Input: part model. Units: mm. Frame: model coordinates. A direction names the side the tool comes from. Coordinates: 2 decimals unless noted, no trailing zeros. Write each loop counter-clockwise with the first axis right and the second up, starting at its lowest first coordinate (ties: lowest second). Pieces come first, ordered by that corner, then holes. Notation, with made-up numbers: M 72,75 L 84,75 A16 ccw 84,105 Z; hole C 55.5,5.25 d10. An arc over 180 degrees is marked long. Write each question's results on one line, items separated by ' | '. Start each with the question number.
1. Ray query, probe 1 along Y at (x, z) = (30, 9.2); probe 2 along Y at (x, z) = (-1.7, 0.8); probe 3 along X at (y, z) = (-19, 0.75). Return the intervals inside material, ascending.
2. Section query A-A, the plane x = 12. Output: boundary loops of the cut face in (y, z).
3. Pull-direction query (Y, two-part tool) for faces 1 (the flat face through (-1, 17, 10)), 2 (the flat face through (0.008, 3.014, 2.571)); classes: +Y half, -Y half, draft (parallel to the pull), parting line (faces both ways), or undercut.
4. Section query C-C, the plane y = -7. Output: boundary loops of the cut face in (x, z).
5. Set-up query: faces 3 (the cylindrical face through (-28.092, -19.399, 8.521)), 4 (the flat face through (-5.164, 0, 3)). Return all of +Z, -Z, +X, -X, +Y, -Y with unobstructed straight access to the full face (end or side cutting, diameter ignored); none if empty.
6. First-contact query: pin 1 (2 mm diameter, centred on x = -13.5, y = -0.5, fed in from +Z); pin 2 (8 mm diameter, centred on x = 35.5, y = -20.5, fed in from -Z); pin 3 (7.5 mm diameter, centred on x = 16, y = -0.5, fed in from +Z). Flat tips, straight axial feed; report the tip coordinate or a pass-through.
7. Section query B-B, the plane y = -20. Output: boundary loops of the cut face in (x, z), and give its area (3 significant figures).
```python
from build123d import *

# Parameters (mm, degrees)
SKETCH_W             = 100
SKETCH_H             = 50
PAD_DEPTH            = 10
SKETCH001_W          = 100
SKETCH001_H          = 18
POCKET_DEPTH         = 1.5
SKETCH002_R          = 2.625
POCKET001_DEPTH      = 8.501
POCKET002_DEPTH      = 7.5
SKETCH004_W          = 77
SKETCH004_H          = 15
PAD001_DEPTH         = 4.5
SKETCH005_R          = 5.25
POCKET003_DEPTH      = 1.2
SKETCH006_R          = 3.5
SKETCH006_R_2        = 2.5
PAD002_DEPTH         = 3
SKETCH008_R          = 2
POCKET005_DEPTH      = 5
SKETCH009_R          = 2
POCKET006_DEPTH      = 5
CHAMFER_SIZE         = 0.49
POCKET007_DEPTH      = 2.15
POCKET007_DEPTH_BACK = 0.85
SKETCH011_R          = 2
POCKET008_DEPTH      = 6
POCKET009_DEPTH      = 3


with BuildPart() as part:
    # Sketch → Pad (new body)
    with BuildSketch(Plane.XY):
        Rectangle(SKETCH_W, SKETCH_H)
    extrude(amount=PAD_DEPTH)

    # Sketch001 (on Face6 of Pad) → Pocket (cut)
    with BuildSketch(Plane.XY.offset(10)):
        Rectangle(SKETCH001_W, SKETCH001_H)
    extrude(amount=-POCKET_DEPTH, mode=Mode.SUBTRACT)

    # Sketch002 (on Face7 of Pocket) → Pocket001 (cut, through all)
    with BuildSketch(Plane.XY.offset(8.5)):
        with Locations((-22.625, 0)):
            Circle(SKETCH002_R)
        with Locations((-12.625, 0)):
            Circle(SKETCH002_R)
        with Locations((-2.625, 0)):
            Circle(SKETCH002_R)
        with Locations((7.375, 0)):
            Circle(SKETCH002_R)
        with Locations((17.375, 0)):
            Circle(SKETCH002_R)
        with Locations((27.375, 0)):
            Circle(SKETCH002_R)
        with Locations((-32.625, 0)):
            Circle(SKETCH002_R)
    extrude(amount=-POCKET001_DEPTH, mode=Mode.SUBTRACT)

    # Sketch003 (on Face4 of Pocket001) → Pocket002 (cut)
    with BuildSketch(Plane(origin=(0, 0, 0), x_dir=(1, 0, 0), z_dir=(0, 0, -1))):
        Polygon((-32.625, -4), (-29.160898, -2), (-29.160898, 2), (-32.625, 4), (-36.089102, 2), (-36.089102, -2), align=None)
        Polygon((-22.625, -4), (-19.160898, -2), (-19.160898, 2), (-22.625, 4), (-26.089102, 2), (-26.089102, -2), align=None)
        Polygon((-12.625, -4), (-9.160898, -2), (-9.160898, 2), (-12.625, 4), (-16.089102, 2), (-16.089102, -2), align=None)
        Polygon((-2.625, -4), (0.839102, -2), (0.839102, 2), (-2.625, 4), (-6.089102, 2), (-6.089102, -2), align=None)
        Polygon((7.375, -4), (10.839102, -2), (10.839102, 2), (7.375, 4), (3.910898, 2), (3.910898, -2), align=None)
        Polygon((17.375, -4), (20.839102, -2), (20.839102, 2), (17.375, 4), (13.910898, 2), (13.910898, -2), align=None)
        Polygon((27.375, -4), (30.839102, -2), (30.839102, 2), (27.375, 4), (23.910898, 2), (23.910898, -2), align=None)
    extrude(amount=-POCKET002_DEPTH, mode=Mode.SUBTRACT)

    # Sketch004 (on DatumPlane) → Pad001 (join)
    with BuildSketch(Plane(origin=(0, 0, 4.5), x_dir=(1, 0, 0), z_dir=(0, 0, -1))):
        Rectangle(SKETCH004_W, SKETCH004_H)
    extrude(amount=PAD001_DEPTH)

    # Sketch005 (on Face4 of Pad001) → Pocket003 (cut)
    with BuildSketch(Plane(origin=(0, 0, 0), x_dir=(1, 0, 0), z_dir=(0, 0, -1))):
        with Locations((38, 20)):
            Circle(SKETCH005_R)
        with Locations((38, -20)):
            Circle(SKETCH005_R)
        with Locations((-1.7, 20)):
            Circle(SKETCH005_R)
        with Locations((-1.7, -20)):
            Circle(SKETCH005_R)
    extrude(amount=-POCKET003_DEPTH, mode=Mode.SUBTRACT)

    # Sketch006 (on Face4 of Pocket003) → Pad002 (join)
    with BuildSketch(Plane(origin=(0, 0, 1.2), x_dir=(1, 0, 0), z_dir=(0, 0, -1))):
        with Locations((-1.7, 0)):
            Circle(SKETCH006_R)
        with Locations((38, 0)):
            Circle(SKETCH006_R_2)
    extrude(amount=PAD002_DEPTH)

    # Sketch008 → Pocket005 (cut)
    with BuildSketch(Plane(origin=(0, 0, -1.8), x_dir=(1, 0, 0), z_dir=(0, 0, -1))):
        with Locations((-1.7, 0)):
            Circle(SKETCH008_R)
        with Locations((38, 0)):
            Circle(SKETCH008_R)
    extrude(amount=-POCKET005_DEPTH, mode=Mode.SUBTRACT)

    # Sketch009 (on Face33 of Pad002) → Pocket006 (cut)
    with BuildSketch(Plane(origin=(0, 0, -1.8), x_dir=(1, 0, 0), z_dir=(0, 0, -1))):
        with Locations((-1.7, 0)):
            Circle(SKETCH009_R)
        with Locations((38, 0)):
            Circle(SKETCH009_R)
    extrude(amount=-POCKET006_DEPTH, mode=Mode.SUBTRACT)

    # Chamfer
    chamfer_edges = [part.edges().sort_by_distance(p)[0] for p in [
        (-5.2, 0, -1.8),
        (35.5, 0, -1.8),
    ]]
    chamfer(chamfer_edges, length=CHAMFER_SIZE)

    # Sketch010 (on Face37 of Chamfer) → Pocket007 (cut, two sides)
    with BuildSketch(Plane(origin=(0, 0, 3.2), x_dir=(1, 0, 0), z_dir=(0, 0, -1))) as pocket007_sk:
        Polygon((-1.7, -4), (1.764102, -2), (1.764102, 2), (-1.7, 4), (-5.164102, 2), (-5.164102, -2), align=None)
        Polygon((34.535898, -2), (38, -4), (41.464102, -2), (41.464102, 2), (38, 4), (34.535898, 2), align=None)
    extrude(amount=POCKET007_DEPTH, mode=Mode.SUBTRACT)
    extrude(pocket007_sk.sketch, amount=-POCKET007_DEPTH_BACK, mode=Mode.SUBTRACT)

    # Sketch011 (on Face33 of Pocket007) → Pocket008 (cut)
    with BuildSketch(Plane.XY.offset(10)):
        with Locations((-30, 20)):
            Circle(SKETCH011_R)
        with Locations((30, 20)):
            Circle(SKETCH011_R)
        with Locations((30, -20)):
            Circle(SKETCH011_R)
        with Locations((-30, -20)):
            Circle(SKETCH011_R)
    extrude(amount=-POCKET008_DEPTH, mode=Mode.SUBTRACT)

    # Sketch012 (on Face66 of Pocket008) → Pocket009 (cut)
    with BuildSketch(Plane.XY.offset(4)):
        Polygon((-30, 16), (-26.535898, 18), (-26.535898, 22), (-30, 24), (-33.464102, 22), (-33.464102, 18), align=None)
        Polygon((30, 16), (33.464102, 18), (33.464102, 22), (30, 24), (26.535898, 22), (26.535898, 18), align=None)
        Polygon((-30, -24), (-26.535898, -22), (-26.535898, -18), (-30, -16), (-33.464102, -18), (-33.464102, -22), align=None)
        Polygon((30, -24), (33.464102, -22), (33.464102, -18), (30, -16), (26.535898, -18), (26.535898, -22), align=None)
    extrude(amount=POCKET009_DEPTH, mode=Mode.SUBTRACT)


solid = part.part
```
Answer:
1) probe 1: -25 to -22, -18 to -9, 9 to 18, 22 to 25 | probe 2: -14.75 to -2, 2 to 14.75 | probe 3: -50 to -6.85, 3.45 to 32.85, 43.15 to 50
2) outline: M -25,0 L 25,0 L 25,10 L 9,10 L 9,8.5 L -9,8.5 L -9,10 L -25,10 Z
3) face 1: draft | face 2: undercut
4) outline: M -50,0 L 50,0 L 50,8.5 L -50,8.5 Z
5) face 3: +Z | face 4: none
6) pin 1: z = 4.5 | pin 2: z = 0 | pin 3: z = 8.5
7) outline: M -50,0 L -6.95,0 L -6.95,1.2 L 3.55,1.2 L 3.55,0 L 32.75,0 L 32.75,1.2 L 43.25,1.2 L 43.25,0 L 50,0 L 50,10 L 32,10 L 32,7 L 33.46,7 L 33.46,4 L 26.54,4 L 26.54,7 L 28,7 L 28,10 L -28,10 L -28,7 L -26.54,7 L -26.54,4 L -33.46,4 L -33.46,7 L -32,7 L -32,10 L -50,10 Z | area: 909 mm^2
